```python
from build123d import *

# Parameters (mm, degrees)
SKETCH1_W                = 8
SKETCH1_H                = 18.5
SKETCH1_R                = 2.25
BOSS_EXTRUDE1_DEPTH      = 5.5
SKETCH1_3_W              = 5.95
SKETCH1_3_H              = 9.5
BOSS_EXTRUDE2_DEPTH      = 9.5
SKETCH1_4_W              = 8
SKETCH1_4_H              = 18.5
SKETCH1_4_R              = 2.25
BOSS_EXTRUDE3_DEPTH      = 5.5
SKETCH1_5_W              = 5.946489343
SKETCH1_5_H              = 9.324210581
BOSS_EXTRUDE4_DEPTH      = 9.5
SKETCH1_6_W              = 5.95
SKETCH1_6_H              = 9.5
SKETCH1_6_W_2            = 5.946489343
SKETCH1_6_H_2            = 9.324210581
BOSS_EXTRUDE5_DEPTH      = 9.5
BOSS_EXTRUDE5_DEPTH_BACK = 45
SKETCH2_R                = 80
BOSS_EXTRUDE6_DEPTH      = 5


with BuildPart() as part:
    # Sketch1 → Boss-Extrude1 (new body)
    with BuildSketch(Plane(origin=(0, 0, 0), x_dir=(1, 0, 0), z_dir=(0, 1, 0))):
        with Locations((-12.015677219, 9.304747116)):
            Rectangle(SKETCH1_W, SKETCH1_H)
        with Locations((-12.009707421, 4.656325954)):
            Circle(SKETCH1_R, mode=Mode.SUBTRACT)
        with Locations((-12.009707421, 14.156325954)):
            Circle(SKETCH1_R, mode=Mode.SUBTRACT)
    extrude(amount=BOSS_EXTRUDE1_DEPTH)

    # Sketch1_3 → Boss-Extrude2 (add)
    with BuildSketch(Plane(origin=(0, 0, 0), x_dir=(1, 0, 0), z_dir=(0, 1, 0))):
        with BuildLine():
            Line((-16.015677219, 0.054747116), (-16.015677219, 18.5))
            Line((-16.015677219, 18.5), (-68.166690169, 18.5))
            ThreePointArc((-68.166690169, 18.5), (-68.959479844, 9.288334925), (-68.486040188, 0.054747116))
            Line((-68.486040188, 0.054747116), (-16.015677219, 0.054747116))
        make_face()
        with Locations((-26.93769232, 9.406325954)):
            Rectangle(SKETCH1_3_W, SKETCH1_3_H, mode=Mode.SUBTRACT)
    extrude(amount=BOSS_EXTRUDE2_DEPTH)



with BuildPart() as body_2:
    # Sketch1_4 → Boss-Extrude3 (new body)
    with BuildSketch(Plane(origin=(0, 0, 0), x_dir=(1, 0, 0), z_dir=(0, 1, 0))):
        with Locations((35.998888009, 9.48618908)):
            Rectangle(SKETCH1_4_W, SKETCH1_4_H)
        with Locations((36.004857807, 4.837767918)):
            Circle(SKETCH1_4_R, mode=Mode.SUBTRACT)
        with Locations((36.004857807, 14.337767918)):
            Circle(SKETCH1_4_R, mode=Mode.SUBTRACT)
    extrude(amount=BOSS_EXTRUDE3_DEPTH)

    # Sketch1_5 → Boss-Extrude4 (add)
    with BuildSketch(Plane(origin=(0, 0, 0), x_dir=(1, 0, 0), z_dir=(0, 1, 0))):
        with BuildLine():
            Line((39.998888009, 18.73618908), (68.768167169, 18.73618908))
            ThreePointArc((68.768167169, 18.73618908), (69.409600563, 9.486508045), (68.777433584, 0.23618908))
            Line((68.777433584, 0.23618908), (39.998888009, 0.23618908))
            Line((39.998888009, 0.23618908), (39.998888009, 18.73618908))
        make_face()
        with Locations((51.410282917, 9.499873209)):
            Rectangle(SKETCH1_5_W, SKETCH1_5_H, mode=Mode.SUBTRACT)
    extrude(amount=BOSS_EXTRUDE4_DEPTH)


with BuildPart() as part_1:
    add(part.part)

    add(body_2.part)  # Boss-Extrude5 merges body 2
    # Sketch1_6 → Boss-Extrude5 (add, two sides)
    with BuildSketch(Plane(origin=(0, 0, 0), x_dir=(1, 0, 0), z_dir=(0, 1, 0))) as boss_extrude5_sk:
        with Locations((-26.93769232, 9.406325954)):
            Rectangle(SKETCH1_6_W, SKETCH1_6_H)
        with Locations((51.410282917, 9.499873209)):
            Rectangle(SKETCH1_6_W_2, SKETCH1_6_H_2)
    extrude(amount=BOSS_EXTRUDE5_DEPTH)
    extrude(boss_extrude5_sk.sketch, amount=-BOSS_EXTRUDE5_DEPTH_BACK)

    # Sketch2 → Boss-Extrude6 (add)
    with BuildSketch(Plane.XZ.offset(45)):
        with Locations((-0.015677219, -9.406325954)):
            Circle(SKETCH2_R)
    extrude(amount=-BOSS_EXTRUDE6_DEPTH)


solid = part_1.part
```
Model file for the job. Use its own axes, mm. A direction names the side the tool comes from. Coordinates: 2 decimals unless noted, no trailing zeros. Order: outer loops, then holes, each group sorted by start corner. A loop starts at its lowest first (then second) coordinate and runs counter-clockwise, first axis right, second up. Notation, with made-up numbers: (62, 27.25) - (96, 27.25) arc R24 cw to (96, 54.25) - close; hole circle Ø4 at (51, 83). An arc over 180 degrees is marked (long way). Return JSON: item names as keys, results as strings. Group by question number.
1) Saw through at B-B, the plane x = 46. Write the cut outline in (y, z).
2) Saw through at A-A, the plane y = -38. Write the cut outline in (x, z).
3) Tool access for faces 4 (the flat face through (-27, -20, -4.656)), 5 (the cylindrical face through (38.15, 2.71, -5.51)), 6 (the flat face through (-42, 5, -18.5)), 7 (the flat face through (48.437, -20, -9)), 8 (the flat face through (31.999, 3, -9)): list every direction of +Z, -Z, +X, -X, +Y, -Y with a clear straight run to the whole face (end or side of a thin tool).
4) Saw through at D-D, the plane z = -30.5. Write the cut outline in (x, y).
5) Saw through at C-C, the plane y = 2. Write the cut outline in (x, z).
6) Flat gauge pins, fed straight in: P1, Ø1, axis at x = 54, y = -19, coming from the +Z side; P2, Ø5, axis at x = -26, y = -26.5, coming from the -Z side; P3, Ø3, axis at x = -26.5, y = -22.5, coming from the +Z side. Where does each tip first touch, or does it go through?
7) Mould opens along X. For faces 1 (the cylindrical face through (-68.957, 4.684, -9.418)), 2 (the flat face through (51, -20, -4.838)), 3 (the flat face through (-8.016, 3, -9)) say: released by +X, released by -X, zero draft, split by the parting line, or undercut.
8) Probe line 1 (Y direction, x = 44.5, z = 21); line 2 (Z direction, x = 62, y = 1); line 3 (X direction, y = -19.5, z = -11). List the from-to ranges inside material, lowest first. Write a range as from..to.
Values found:
{
 "1": {"outline": "(-45, -74.85) - (-40, -74.85) - (-40, 56.03) - (-45, 56.03) - close; (0, -18.74) - (9.5, -18.74) - (9.5, -0.24) - (0, -0.24) - close"},
 "2": {"outline": "(-29.91, -14.16) - (-23.96, -14.16) - (-23.96, -4.66) - (-29.91, -4.66) - close; (48.44, -14.16) - (54.38, -14.16) - (54.38, -4.84) - (48.44, -4.84) - close"},
 "3": {"face 4": "+Z, +X, -X", "face 5": "+Y", "face 6": "-Z, -X, +Y", "face 7": "+Z, -Z", "face 8": "+Z, -Z, +Y"},
 "4": {"outline": "(-77.18, -45) - (77.15, -45) - (77.15, -40) - (-77.18, -40) - close"},
 "5": {"outline": "(-68.49, -0.05) arc R67.5 ccw to (-68.17, -18.5) - (-16.02, -18.5) - (-16.02, -18.55) - (-8.02, -18.55) - (-8.02, -0.05) - close; (32, -18.74) - (68.77, -18.74) arc R67.5 ccw to (68.78, -0.24) - (32, -0.24) - close; hole circle Ø4.5 at (-12.01, -14.16); hole circle Ø4.5 at (-12.01, -4.66); hole circle Ø4.5 at (36, -14.34); hole circle Ø4.5 at (36, -4.84)"},
 "6": {"P1": "stops at z = -4.84", "P2": "stops at z = -14.16", "P3": "stops at z = -4.66"},
 "7": {"face 1": "released by -X", "face 2": "zero draft", "face 3": "undercut"},
 "8": {"line 1": "y = -45..-40", "line 2": "z = -18.74..-0.24", "line 3": "x = -29.91..-23.96, 48.44..54.38"}
}
